The model under review builds one solid part; all positions refer to its coordinate system, in mm. Face numbers are marked on the shaded views. A direction names the side the tool comes from. Round coordinates to 2 decimals unless told otherwise and drop trailing zeros. Loops run counter-clockwise (first coordinate to the right, second up) from the corner with the lowest first, then second, coordinate; pieces in that order, holes last. Notation, with made-up numbers: M -8.75,24.25 L 17.25,24.25 A15 ccw 17.25,34.25 Z; hole C -13,-34.5 d2. An arc over 180 degrees is marked long. Answer in a Markdown table with one row per item. Add a question column.
from build123d import *

# Parameters (mm, degrees)
SKETCH2_R               = 4
SKETCH2_R_2             = 3
BOSS_EXTRUDE1_DEPTH     = 10
CUT_EXTRUDE1_DEPTH      = 45.72135955
CUT_EXTRUDE1_DEPTH_BACK = 45.72135955
SKETCH3_R               = 1.5
SKETCH3_R_2             = 2
SKETCH4_W               = 20
SKETCH4_H               = 45
CUT_EXTRUDE2_DEPTH      = 10


with BuildPart() as part:
    # Sketch1 → Revolve1 (revolve)
    with BuildSketch(Plane.XY, mode=Mode.PRIVATE) as revolve1_sk:
        Polygon((3, 0), (4, 0), (4, 14), (20, 14), (20, 22), (0, 22), (0, 13), (3, 13), align=None)
    revolve(revolve1_sk.sketch.rotate(Axis((0, 0, 0), (0, 1, 0)), 90), axis=Axis((0, 0, 0), (0, 1, 0)))

    # Sketch2 → Boss-Extrude1 (add)
    with BuildSketch(Plane(origin=(0, 22, 0), x_dir=(1, 0, 0), z_dir=(0, 1, 0))):
        with Locations(Location((0, 0, 0), (0, 0, 90))):
            Circle(SKETCH2_R)
        with Locations(Location((0, 0, 0), (0, 0, 90))):
            Circle(SKETCH2_R_2, mode=Mode.SUBTRACT)
    extrude(amount=BOSS_EXTRUDE1_DEPTH)

    # Sketch3 → Cut-Extrude1 (cut, two sides: drawn at the far end of the back side and taken through both)
    with BuildSketch(Plane(origin=(0, 0, -4), x_dir=(-1, 0, 0), z_dir=(0, 0, -1)).offset(-CUT_EXTRUDE1_DEPTH_BACK)):
        with Locations((0, 5)):
            Circle(SKETCH3_R)
        with Locations((0, 27)):
            Circle(SKETCH3_R)
        with Locations((0, 18)):
            Circle(SKETCH3_R_2)
    extrude(amount=CUT_EXTRUDE1_DEPTH + CUT_EXTRUDE1_DEPTH_BACK, mode=Mode.SUBTRACT)

    # Sketch4 → Cut-Extrude2 (cut)
    with BuildSketch(Plane.XZ.offset(-14)):
        with Locations((-20, 0)):
            Rectangle(SKETCH4_W, SKETCH4_H)
        with Locations((20, 0)):
            Rectangle(SKETCH4_W, SKETCH4_H)
    extrude(amount=-CUT_EXTRUDE2_DEPTH, mode=Mode.SUBTRACT)


solid = part.part
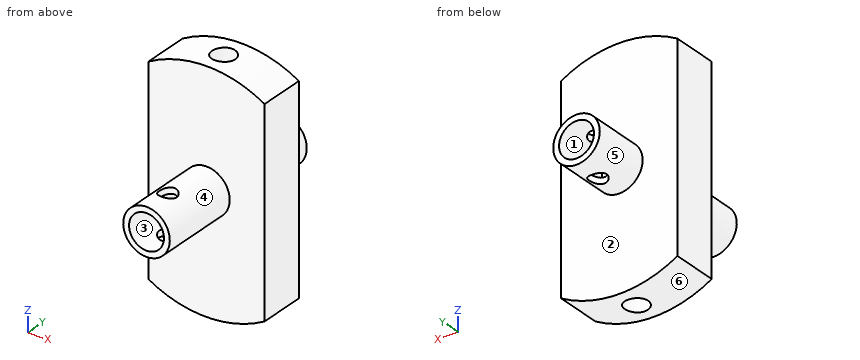
1. Mouldability with a two-part tool opening along Z and no side actions: class the marked faces 1, 2, 3 and 4 as released by +Z, released by -Z, zero draft, split by the parting line, or undercut.
2. Take a section at A-A, the plane y = 18. State the section outline as (x, z) points.
3. For pin 1 Ø12 at (x, y) = (-7, 4) entering from -Z; pin 2 Ø5.5 at (x, z) = (0, 0) entering from -Y; pin 3 Ø4 at (x, y) = (-4, 14.5) entering from +Z, all flat-tipped, find the tip position at first contact; note any pin that passes through.
4. Take a section at D-D, the plane y = 29. State the section outline as (x, z) points.
5. Take a section at C-C, the plane x = 0. State how many separate pieces and enclosed holes the cut face has, and give its area (3 significant figures).
6. Machinability: for the marked faces 5 and 6, which of the approach directions +Z, -Z, +X, -X, +Y, -Y give a long, thin tool a straight path to every point of the face, cutting with its end or side? Answer none if there is none.
7. To check wall thickness, follow probe 1 along Y at (x, z) = (0, 3.2); probe 2 along X at (y, z) = (28.25, 0); probe 3 along Y at (x, z) = (8.25, -1.5). State the ranges of each line that lie inside material, in increasing order.
8. Take a section at B-B, the plane z = -12. State the section outline as (x, y) points.
Check sheet entries:
| question | item | result |
|---|---|---|
| 1 | face 1 | undercut |
| 1 | face 2 | zero draft |
| 1 | face 3 | undercut |
| 1 | face 4 | split by the parting line |
| 2 | outline | M -10,-17.32 A20 ccw -2,-19.9 L -2,19.9 A20 ccw -10,17.32 Z; M 2,-19.9 A20 ccw 10,-17.32 L 10,17.32 A20 ccw 2,19.9 Z |
| 3 | pin 1 | stops at z = -3.87 |
| 3 | pin 2 | stops at y = 13 |
| 3 | pin 3 | stops at z = 19.9 |
| 4 | outline | C 0,0 d8; hole C 0,0 d6 |
| 5 | separate pieces | 6 |
| 5 | enclosed holes | 0 |
| 5 | area | 202 mm^2 |
| 6 | face 5 | +Y |
| 6 | face 6 | -Z, +Y, -Y |
| 7 | probe 1 | y = 0 to 3.5, 6.5 to 16, 20 to 25.5, 28.5 to 32 |
| 7 | probe 2 | x = -4 to -3, 3 to 4 |
| 7 | probe 3 | y = 14 to 22 |
| 8 | outline | M -10,14 L 10,14 L 10,22 L -10,22 Z; hole C 0,18 d4 |
